The figure shows three views and two pictorial views of one solid part (mm, origin at its lowest corner). Answer the questions. Round coordinates to 2 decimals unless told otherwise and drop trailing zeros. Write each loop counter-clockwise with the first axis right and the second up, starting at its lowest first coordinate (ties: lowest second). Pieces come first, ordered by that corner, then holes. Notation, with made-up numbers: M -4.5,18.25 L 29.5,18.25 A28 ccw 29.5,52.25 Z; hole C 11,47 d7. An arc over 180 degrees is marked long. Answer in a Markdown table with one row per item.
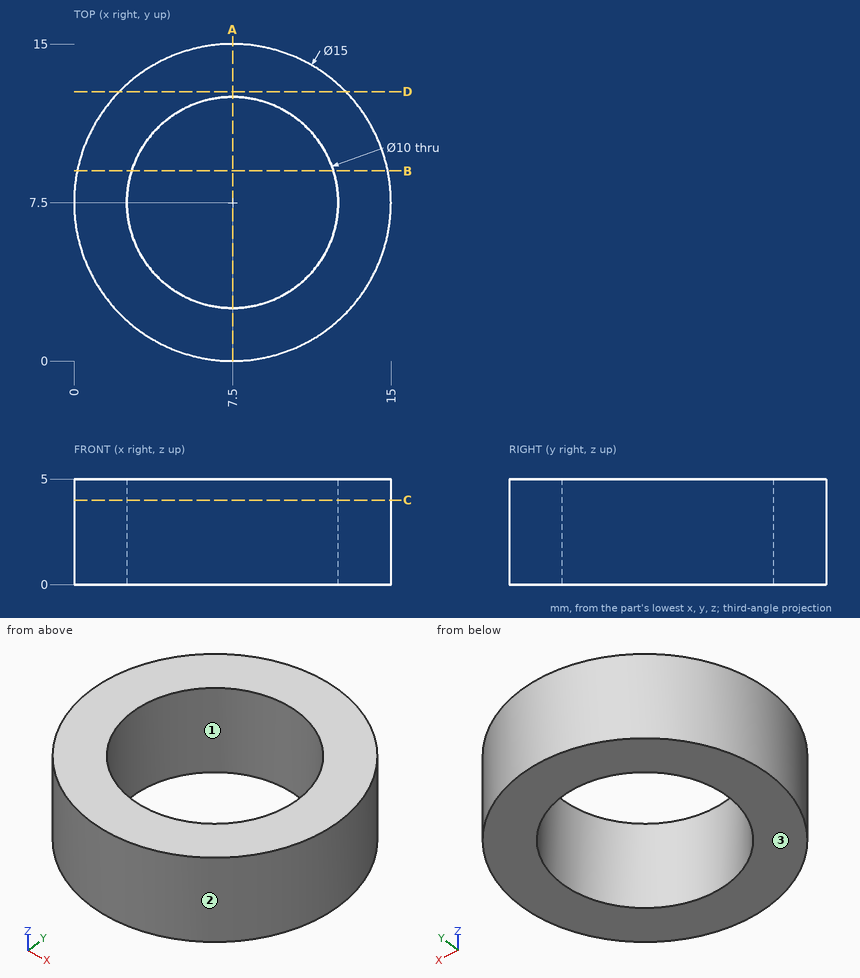
1. The part is cut by section D-D (y = 12.75). Determine the outline of the cut face in (x, z), plus the area to 3 significant figures.
Calculated:
| item | result |
|---|---|
| outline | M 2.14,0 L 12.86,0 L 12.86,5 L 2.14,5 Z |
| area | 53.6 mm² |
2. The part is cut by section B-B (y = 9). Determine the outline of the cut face in (x, z).
Calculated:
| item | result |
|---|---|
| outline | M 0.15,0 L 2.73,0 L 2.73,5 L 0.15,5 Z; M 12.27,0 L 14.85,0 L 14.85,5 L 12.27,5 Z |
3. Given pin 1 (2 mm diameter, centred on y = 12, z = 4.5, fed in from -X); pin 2 (2 mm diameter, centred on x = 10.5, y = 6.5, fed in from +Z), each flat-ended and moving along its own axis, determine where each tip first touches the part or whether it passes through.
Calculated:
| item | result |
|---|---|
| pin 1 | stops at x = 0.87 |
| pin 2 | passes through |
4. Determine the mould class of the marked faces 1, 2 and 3 for opening direction Y: released by +Y, released by -Y, zero draft, split by the parting line, or undercut.
Calculated:
| item | result |
|---|---|
| face 1 | undercut |
| face 2 | split by the parting line |
| face 3 | zero draft |
5. Consider line 1 along Y through (x, z) = (7.5, 1.45); line 2 along X through (y, z) = (4.25, 4.55). Determine where each line is inside the solid, lowest interval first. Write a range as from..to.
Calculated:
| item | result |
|---|---|
| line 1 | y = 0..2.5, 12.5..15 |
| line 2 | x = 0.74..3.7, 11.3..14.26 |
6. The part is cut by section A-A (x = 7.5). Determine the outline of the cut face in (y, z), plus the area to 3 significant figures.
Calculated:
| item | result |
|---|---|
| outline | M 0,0 L 2.5,0 L 2.5,5 L 0,5 Z; M 12.5,0 L 15,0 L 15,5 L 12.5,5 Z |
| area | 25.0 mm² |
7. The part is cut by section C-C (z = 4). Determine the outline of the cut face in (x, y).
Calculated:
| item | result |
|---|---|
| outline | C 7.5,7.5 d15; hole C 7.5,7.5 d10 |
